Geometry: final body of the model. Coordinates: model frame, mm. A direction names the side the tool comes from. Coordinates: 2 decimals unless noted, no trailing zeros. Write each loop counter-clockwise with the first axis right and the second up, starting at its lowest first coordinate (ties: lowest second). Pieces come first, ordered by that corner, then holes. Notation, with made-up numbers: (22, -1.75) - (67, -1.75) arc R3 ccw to (67, 2.25) - close; hole circle Ø11 at (-16, 22.5). An arc over 180 degrees is marked (long way). Put each result on its own line as item: value.
```python
from build123d import *

# Parameters (mm, degrees)
BOSS_EXTRUDE1_DEPTH = 25.4
SKETCH2_R           = 3.175
CUT_EXTRUDE1_DEPTH  = 4.175
FILLET1_R           = 2.54


with BuildPart() as part:
    # Sketch1 → Boss-Extrude1 (new body)
    with BuildSketch(Plane(origin=(0, 0, 0), x_dir=(0, 0, -1), z_dir=(1, 0, 0))):
        with BuildLine():
            Line((0, 0), (-21.997045256, 12.7))
            Line((-21.997045256, 12.7), (-23.584545256, 9.950369343))
            Line((-23.584545256, 9.950369343), (-1.5875, -2.749630657))
            ThreePointArc((-1.5875, -2.749630657), (-0.821750468, -3.066814498), (0, -3.175))
            Line((0, -3.175), (393.7, -3.175))
            Line((393.7, -3.175), (393.7, 0))
            Line((393.7, 0), (0, 0))
        make_face()
    extrude(amount=BOSS_EXTRUDE1_DEPTH)

    # Sketch2 → Cut-Extrude1 (cut, through all)
    with BuildSketch(Plane(origin=(0, 0, 0), x_dir=(1, 0, 0), z_dir=(0, 1, 0))):
        with Locations((12.7, 88.9)):
            Circle(SKETCH2_R)
        with Locations((12.7, 304.8)):
            Circle(SKETCH2_R)
    extrude(amount=-CUT_EXTRUDE1_DEPTH, mode=Mode.SUBTRACT)

    # Fillet1
    fillet1_edges = [part.edges().sort_by_distance(p)[0] for p in [
        (25.4, 11.325184671, 22.790795256),
        (12.7, 0, 0),
        (25.4, -1.5875, -393.7),
        (0, -1.5875, -393.7),
        (0, 11.325184671, 22.790795256),
    ]]
    fillet(fillet1_edges, radius=FILLET1_R)


solid = part.part
```
1. Section query C-C (y = 3.75). Return loops of the section in (x, z).
Answer below:
outline: (0, 6.5) - (25.4, 6.5) - (25.4, 12.85) - (0, 12.85) - close
2. Set-up query: faces 1 (the flat face through (13, 0, -200)), 2 (the flat face through (0, -1, -184)). Return all of +Z, -Z, +X, -X, +Y, -Y with unobstructed straight access to the full face (end or side cutting, diameter ignored); none if empty.
Answer below:
face 1: -Z, +X, -X, +Y
face 2: +Z, -Z, -X, +Y, -Y
3. Section query B-B (z = -111.5). Return loops of the section in (x, y) (3 decimals), then the cut area to 3 significant figures.
Answer below:
outline: (0, -3.175) - (25.4, -3.175) - (25.4, 0) - (0, 0) - close
area: 80.6 mm²
4. Pin query (flat end, axial travel): pin 1 Ø4 at (x, y) = (7.5, 11) entering from +Z; pin 2 Ø6 at (y, z) = (4, -179) entering from +X; pin 3 Ø1 at (x, z) = (9.5, -18.5) entering from +Y; pin 4 Ø2 at (x, y) = (20.5, 7) entering from -Z. Return the tip coordinate at first contact, or that it passes through.
Answer below:
pin 1: stops at z = 23.58
pin 2: passes through
pin 3: stops at y = 0
pin 4: stops at z = 10.39
5. Ray query, probe 1 along X at (y, z) = (-1.1, -304.8) (3 decimals); probe 2 along Z at (x, y) = (12.7, -2.25) (3 decimals); probe 3 along Z at (x, y) = (12.7, -0.7) (3 decimals). Return the intervals inside material, ascending. Write a range as from..to.
Answer below:
probe 1: x = 0..9.525, 15.875..25.4
probe 2: z = -393.7..-307.975, -301.625..-92.075, -85.725..2.453
probe 3: z = -393.7..-307.975, -301.625..-92.075, -85.725..5.138
6. Mould query, pull axis X, two halves, no side actions, for faces 3 (the flat face through (13, -3.175, -194)), 4 (the cylindrical face through (12.01, -1.57, -301.7)), 5 (the flat face through (25.4, -1, -184)). Classes: +X half, -X half, draft (parallel to the pull), parting line (faces both ways), or undercut.
Answer below:
face 3: draft
face 4: undercut
face 5: +X half
